Input: part model. Units: mm. Frame: model coordinates. Coordinates: 2 decimals unless noted, no trailing zeros. Order: outer loops, then holes, each group sorted by start corner. A loop starts at its lowest first (then second) coordinate and runs counter-clockwise, first axis right, second up.
from build123d import *

# Parameters (mm, degrees)
SKETCH_1_W          = 74
SKETCH_1_H          = 55
EXTRUDE_1_DEPTH     = 3
SKETCH_2_R          = 1.6
CUT_EXTRUDE_1_DEPTH = 4
SKETCH_2_3_R        = 1.3
CUT_EXTRUDE_2_DEPTH = 4


with BuildPart() as part:
    # 草圖1 → 填料-伸長1 (new body)
    with BuildSketch(Plane.XY):
        Rectangle(SKETCH_1_W, SKETCH_1_H)
    extrude(amount=EXTRUDE_1_DEPTH)

    # 草圖2 → 除料-伸長1 (cut, through all)
    with BuildSketch(Plane.XY.offset(3)):
        with Locations((-33.55, 0)):
            Circle(SKETCH_2_R)
        with Locations((33.55, 0)):
            Circle(SKETCH_2_R)
        with Locations((-23, 0)):
            Circle(SKETCH_2_R)
        with Locations((23, 0)):
            Circle(SKETCH_2_R)
    extrude(amount=-CUT_EXTRUDE_1_DEPTH, mode=Mode.SUBTRACT)

    # 草圖2<3> → 除料-伸長2 (cut, through all)
    with BuildSketch(Plane.XY.offset(3)):
        with Locations((16.5, 0)):
            Circle(SKETCH_2_3_R)
        with Locations((14.449747468, -4.949747468)):
            Circle(SKETCH_2_3_R)
        with Locations((9.5, -7)):
            Circle(SKETCH_2_3_R)
        with Locations((4.550252532, -4.949747468)):
            Circle(SKETCH_2_3_R)
        with Locations((2.5, 0)):
            Circle(SKETCH_2_3_R)
        with Locations((4.550252532, 4.949747468)):
            Circle(SKETCH_2_3_R)
        with Locations((9.5, 7)):
            Circle(SKETCH_2_3_R)
        with Locations((14.449747468, 4.949747468)):
            Circle(SKETCH_2_3_R)
    extrude(amount=-CUT_EXTRUDE_2_DEPTH, mode=Mode.SUBTRACT)


solid = part.part
Item 1: Draft query along X for faces 1 (the face through (-1, 0, 3)), 2 (the face through (14.17, -6.22, 1.52)), 3 (the face through (-37, 0, 1)). Return one class per face: pulls with the +X half, pulls with the -X half, needs draft (parallel to the pull), parting line crosses it, or undercut.
Response values:
face 1: needs draft
face 2: undercut
face 3: pulls with the -X half
Item 2: Cut plane B-B on y = -7. Return loops of the section in (x, z), then the cut area to 3 significant figures.
Response values:
outline: (-37, 0) - (8.2, 0) - (8.2, 3) - (-37, 3) - close; (10.8, 0) - (37, 0) - (37, 3) - (10.8, 3) - close
area: 214 mm2
Item 3: Ray query, probe 1 along X at (y, z) = (5, 1.6); probe 2 along Y at (x, z) = (16.5, 0.9); probe 3 along Y at (x, z) = (23, 1.35). Return the intervals inside material, ascending.
Response values:
probe 1: x = -37 to 3.25, 5.85 to 13.15, 15.75 to 37
probe 2: y = -27.5 to -1.3, 1.3 to 27.5
probe 3: y = -27.5 to -1.6, 1.6 to 27.5
Item 4: Cut plane C-C on z = 1.7. Count the separate pieces of the cut face and the enclosed holes in it, then the cut area to 3 significant figures.
Response values:
separate pieces: 1
enclosed holes: 12
area: 4,000 mm2
Item 5: Cut plane A-A on x = 16.5. Return loops of the section in (y, z).
Response values:
outline: (-27.5, 0) - (-1.3, 0) - (-1.3, 3) - (-27.5, 3) - close; (1.3, 0) - (27.5, 0) - (27.5, 3) - (1.3, 3) - close
Item 6: Pin query (flat end, axial travel): pin 1 Ø2.5 at (x, y) = (14.45, 4.95) entering from +Z. Return the tip coordinate at first contact, or that it passes through.
Response values:
pin 1: passes through
